Could you check a few things on this model? Use its own coordinates, in mm. A direction names the side the tool comes from. Round coordinates to 2 decimals unless told otherwise and drop trailing zeros. Write each loop counter-clockwise with the first axis right and the second up, starting at its lowest first coordinate (ties: lowest second). Pieces come first, ordered by that corner, then holes. Notation, with made-up numbers: M 64,1.25 L 83,1.25 A12 ccw 83,10.25 Z; hole C -23,-39.75 d10. An arc over 180 degrees is marked long. One line per item, written item: value. Start each with the question number.
(1) I'm going to push flat-ended pins straight in: pin 1 Ø8 at (x, y) = (9, 89) entering from +Z; pin 2 Ø10 at (x, y) = (2.5, 79) entering from +Z; pin 3 Ø2 at (y, z) = (27, 0.5) entering from +X; pin 4 Ø3 at (y, z) = (61.5, 1) entering from -X. Where does each tip first touch, or does it pass through?
(2) Which directions (+Z, -Z, +X, -X, +Y, -Y) give clear straight access to the entire face, cutting with the end or side of a thin tool? Please do faces 4 (the face through (-16, 49, 2.75)), 5 (the face through (0.33, 97.48, -3.26)), 6 (the face through (13.5, 49, -1)), 7 (the face through (-12.5, 49, 0)), 8 (the face through (15, 49, 3.75)).
(3) I want a section at B-B on z = -0.75. Please give me the cut outline in (x, y).
(4) I want a section at C-C on y = 47. Please give me the cut outline in (x, z).
(5) Thinking about a two-plate mould opening in X: for faces 1 (the face through (-13.5, 49, 0)), 2 (the face through (0.33, 7.48, -3.26)), 3 (the face through (0, 100, -3)), which applies, released by +X, released by -X, zero draft, split by the parting line, or undercut?
(6) I want a section at D-D on y = 95. Please give me the cut outline in (x, z), and give its area (3 significant figures).
(7) I want a section at A-A on x = 0. Please give me the cut outline in (y, z), and give its area (3 significant figures).
(8) If I drill on L1, parallel to Y at x = 0, z = -3.25; L2, parallel to X at y = 67.5, z = 1; L3, parallel to Z at x = 1, y = 52.5, over which ranges is the centre line in solid material (lowest first)?
```python
from build123d import *

# Parameters (mm, degrees)
F1_DEPTH = 100
F3_D     = 5


with BuildPart() as f1:
    # F0 (on Front) → F1 (new body)
    with BuildSketch(Plane.XZ):
        Polygon((-12.5, 3.75), (-17.5, 3.75), (-17.5, 2.75), (-13.5, 2.75), (-13.5, -3.75), (-2.6, -3.75), (2.6, -3.75), (13.5, -3.75), (13.5, 2.75), (17.5, 2.75), (17.5, 3.75), (12.5, 3.75), (12.5, -2.75), (2.6, -2.75), (-2.6, -2.75), (-12.5, -2.75), align=None)
    extrude(amount=-F1_DEPTH)

    # F3 (through all)
    with Locations(Plane.XY.offset(-2.75)):
        with Locations((0, 95), (0, 5)):
            Hole(F3_D / 2)


solid = f1.part
```
Found:
1. pin 1: stops at z = 3.75
1. pin 2: stops at z = -2.75
1. pin 3: stops at x = 13.5
1. pin 4: stops at x = -13.5
2. face 4: -Z, -X, +Y, -Y
2. face 5: +Z, -Z
2. face 6: -Z, +X, +Y, -Y
2. face 7: +Z, +Y, -Y
2. face 8: +Z, +X, -X, +Y, -Y
3. outline: M -13.5,0 L -12.5,0 L -12.5,100 L -13.5,100 Z; M 12.5,0 L 13.5,0 L 13.5,100 L 12.5,100 Z
4. outline: M -17.5,2.75 L -13.5,2.75 L -13.5,-3.75 L 13.5,-3.75 L 13.5,2.75 L 17.5,2.75 L 17.5,3.75 L 12.5,3.75 L 12.5,-2.75 L -12.5,-2.75 L -12.5,3.75 L -17.5,3.75 Z
5. face 1: released by -X
5. face 2: undercut
5. face 3: zero draft
6. outline: M -17.5,2.75 L -13.5,2.75 L -13.5,-3.75 L -2.5,-3.75 L -2.5,-2.75 L -12.5,-2.75 L -12.5,3.75 L -17.5,3.75 Z; M 2.5,-3.75 L 13.5,-3.75 L 13.5,2.75 L 17.5,2.75 L 17.5,3.75 L 12.5,3.75 L 12.5,-2.75 L 2.5,-2.75 Z
6. area: 43.0 mm²
7. outline: M 0,-3.75 L 2.5,-3.75 L 2.5,-2.75 L 0,-2.75 Z; M 7.5,-3.75 L 92.5,-3.75 L 92.5,-2.75 L 7.5,-2.75 Z; M 97.5,-3.75 L 100,-3.75 L 100,-2.75 L 97.5,-2.75 Z
7. area: 90.0 mm²
8. L1: y = 0 to 2.5, 7.5 to 92.5, 97.5 to 100
8. L2: x = -13.5 to -12.5, 12.5 to 13.5
8. L3: z = -3.75 to -2.75
